Build history of the part. All positions in model axes, mm. A direction names the side the tool comes from. Round coordinates to 2 decimals unless told otherwise and drop trailing zeros. Write each loop counter-clockwise with the first axis right and the second up, starting at its lowest first coordinate (ties: lowest second). Pieces come first, ordered by that corner, then holes.
1) Saw through at D-D (x = -17). Write the cut outline in (y, z).
2) Pull direction Z, two halves, no side cores. Call faces 6 (the flat face through (7, 5, -12.7)), 7 (the cylindrical face through (6.091, 1.476, 18.406)), 8 (the cylindrical face through (4.354, 5.339, -5.795)): +Z half, -Z half, draft (parallel to the pull), parting line (faces both ways), or undercut.
3) Saw through at C-C (z = 8.5). Write the cut outline in (x, y), plus the area to 3 significant figures.
4) Flat gauge pins, fed straight in: pin 1 (9.5 mm diameter, centred on x = -12, y = 5.5, fed in from -Z); pin 2 (0.5 mm diameter, centred on x = 9, z = 9, fed in from +Y); pin 3 (4 mm diameter, centred on y = 4.5, z = 12, fed in from +X). Where does each tip first touch, or does it go through?
5) Wall check: probe 1 along Z at (x, y) = (-18, -3); probe 2 along Y at (x, z) = (6, 12); probe 3 along Y at (x, z) = (9.5, 2.5). Give the ranges that are in metal, low to high.
6) Which spindle directions (+Z, -Z, +X, -X, +Y, -Y) get a long thin tool onto all of the face, cutting with end or side? Do faces 1 (the flat face through (8, 7, 17.78)), 2 (the cylindrical face through (6.091, 1.476, -12.074)), 3 (the flat face through (7, 5, 19.05)), 4 (the flat face through (9.455, 4, 11)), 5 (the cylindrical face through (16.22, 4.74, 3.13)). Say none if no direction does.
7) Saw through at B-B (z = 3.5). Write the cut outline in (x, y) (3 decimals), plus the area to 3 significant figures.
8) Saw through at A-A (x = -72). Write the cut outline in (y, z).
from build123d import *

# Parameters (mm, degrees)
SKETCH1_R                = 6.35
BOSS_EXTRUDE1_DEPTH      = 6.35
BOSS_EXTRUDE2_DEPTH      = 12.7
BOSS_EXTRUDE2_DEPTH_BACK = 19.05
SKETCH2_R                = 3.175
CUT_EXTRUDE1_START       = -1.27
SKETCH9_OUTSIDE_W        = 125.228
SKETCH9_OUTSIDE_H        = 42.678
SKETCH9_OUTSIDE_R        = 2.547934527
CUT_EXTRUDE1_DEPTH       = 11.43
CUT_EXTRUDE2_START       = -1.27
SKETCH10_OUTSIDE_W       = 125.228
SKETCH10_OUTSIDE_H       = 42.678
SKETCH10_OUTSIDE_R       = 2.542549773
CUT_EXTRUDE2_DEPTH       = 11.43
SKETCH11_W               = 0.667064712
SKETCH11_H               = 3.541255891
BOSS_EXTRUDE3_DEPTH      = 10.16


with BuildPart() as part:
    # Sketch1 → Boss-Extrude1 (new body)
    with BuildSketch(Plane.XY):
        with BuildLine():
            Line((-75.85152439, 14.055182927), (6.69847561, 14.055182927))
            ThreePointArc((6.69847561, 14.055182927), (16.22347561, 4.530182927), (6.69847561, -4.994817073))
            Line((6.69847561, -4.994817073), (-75.85152439, -4.994817073))
            ThreePointArc((-75.85152439, -4.994817073), (-85.37652439, 4.530182927), (-75.85152439, 14.055182927))
        make_face()
        with Locations((-75.85152439, 4.530182927)):
            Circle(SKETCH1_R, mode=Mode.SUBTRACT)
    extrude(amount=BOSS_EXTRUDE1_DEPTH)

    # Sketch2 → Boss-Extrude2 (add, two sides: drawn at the far end of the back side and taken through both)
    with BuildSketch(Plane.XY.offset(6.35).offset(-BOSS_EXTRUDE2_DEPTH_BACK)):
        with Locations((6.779432591, 4.575242679)):
            Circle(SKETCH2_R)
    extrude(amount=BOSS_EXTRUDE2_DEPTH + BOSS_EXTRUDE2_DEPTH_BACK)

    # Sketch9 outside → Cut-Extrude1 (cut)
    with BuildSketch(Plane.XY.offset(19.05).offset(CUT_EXTRUDE1_START)):
        with Locations((-34.577, 4.53)):
            Rectangle(SKETCH9_OUTSIDE_W, SKETCH9_OUTSIDE_H)
        with Locations((6.779432591, 4.575242679)):
            Circle(SKETCH9_OUTSIDE_R, mode=Mode.SUBTRACT)
    extrude(amount=-CUT_EXTRUDE1_DEPTH, mode=Mode.SUBTRACT)

    # Sketch10 outside → Cut-Extrude2 (cut)
    with BuildSketch(Plane(origin=(0, 0, -12.7), x_dir=(-1, 0, 0), z_dir=(0, 0, -1)).offset(CUT_EXTRUDE2_START)):
        with Locations((34.577, 4.53)):
            Rectangle(SKETCH10_OUTSIDE_W, SKETCH10_OUTSIDE_H)
        with Locations((-6.779432591, 4.575242679)):
            Circle(SKETCH10_OUTSIDE_R, mode=Mode.SUBTRACT)
    extrude(amount=-CUT_EXTRUDE2_DEPTH, mode=Mode.SUBTRACT)

    # Sketch11 → Boss-Extrude3 (add)
    with BuildSketch(Plane.XY.offset(6.35)):
        with Locations((9.121178525, 4.372750116)):
            Rectangle(SKETCH11_W, SKETCH11_H)
    extrude(amount=BOSS_EXTRUDE3_DEPTH)


solid = part.part
Evaluation:
1. outline: (-4.99, 0) - (14.06, 0) - (14.06, 6.35) - (-4.99, 6.35) - close
2. face 6: -Z half
2. face 7: draft
2. face 8: undercut
3. outline: (8.79, 2.6) - (9.45, 2.6) - (9.45, 6.14) - (8.79, 6.14) arc R2.55 ccw (long way) to (8.79, 3.01) - close
3. area: 21.6 mm2
4. pin 1: stops at z = 0
4. pin 2: stops at y = 6.19
4. pin 3: stops at x = 9.45
5. probe 1: z = 0 to 6.35
5. probe 2: y = 2.15 to 7
5. probe 3: y = -4.57 to 13.63
6. face 1: none
6. face 2: -Z
6. face 3: +Z, +X, -X, +Y, -Y
6. face 4: +X, +Y, -Y
6. face 5: +Z, -Z, +X
7. outline: (-75.852, -4.995) - (6.698, -4.995) arc R9.525 ccw to (6.698, 14.055) - (-75.852, 14.055) arc R9.525 ccw to start; hole circle Ø12.7 at (-75.852, 4.53)
7. area: 1,730 mm2
8. outline: (-4.99, 0) - (-0.52, 0) - (-0.52, 6.35) - (-4.99, 6.35) - close; (9.58, 0) - (14.06, 0) - (14.06, 6.35) - (9.58, 6.35) - close
